Design review of the part built by this model. Coordinates are the model's own, in mm. Face numbers are marked on the shaded views. A direction names the side the tool comes from. Give positions to 0.01 mm unless a question says otherwise; leave off trailing zeros. Write each loop counter-clockwise with the first axis right and the second up, starting at its lowest first coordinate (ties: lowest second). Pieces come first, ordered by that corner, then holes. Notation, with made-up numbers: (51, -16.75) -> (66, -16.75) arc R15 ccw to (66, -5.75) -> close; hole circle Ø5 at (-4, -30.75). An arc over 180 degrees is marked (long way). Answer as a JSON object with one key per item and string values.
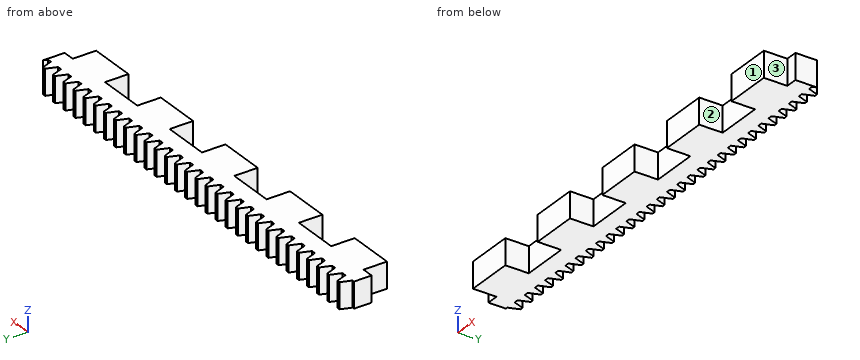
```python
from build123d import *

# Parameters (mm, degrees)
BLANKSKE_W          = 95
BLANKSKE_H          = 11
BLANK_DEPTH         = 5.5
TOOTHCUTSIM_DEPTH   = 96.792745028
TEETHCUTS_COUNT     = 31
TEETHCUTS_PITCH     = 3.14159265
SKETCH_1_W          = 10
SKETCH_1_H          = 5
CUT_EXTRUDE_1_DEPTH = 96.792745028


with BuildPart() as part:
    # BlankSke → Blank (new body)
    with BuildSketch(Plane.XY):
        with Locations((47.5, 5.5)):
            Rectangle(BLANKSKE_W, BLANKSKE_H)
    extrude(amount=-BLANK_DEPTH)

    # TooCutSkeSim → ToothCutSim (cut, through all)
    with BuildSketch(Plane.XY):
        Polygon((0.44443537, 8.75), (-0.44443537, 8.75), (-1.272613241, 11.0254), (1.272613241, 11.0254), align=None)
    toothcutsim = extrude(amount=-TOOTHCUTSIM_DEPTH, mode=Mode.SUBTRACT)

    # TeethCuts: ToothCutSim ×31
    with Locations(*[(i * TEETHCUTS_PITCH, 0, 0) for i in range(1, TEETHCUTS_COUNT)]):
        add(toothcutsim, mode=Mode.SUBTRACT)

    # ｽｹｯﾁ1 → ｶｯﾄ - 押し出し1 (cut, through all)
    with BuildSketch(Plane.XY):
        with Locations((-2.5, 2.5)):
            Rectangle(SKETCH_1_W, SKETCH_1_H)
        with Locations((17.5, 2.5)):
            Rectangle(SKETCH_1_W, SKETCH_1_H)
        with Locations((37.5, 2.5)):
            Rectangle(SKETCH_1_W, SKETCH_1_H)
        with Locations((57.5, 2.5)):
            Rectangle(SKETCH_1_W, SKETCH_1_H)
        with Locations((77.5, 2.5)):
            Rectangle(SKETCH_1_W, SKETCH_1_H)
        with Locations((97.5, 2.5)):
            Rectangle(SKETCH_1_W, SKETCH_1_H)
    extrude(amount=-CUT_EXTRUDE_1_DEPTH, mode=Mode.SUBTRACT)


solid = part.part
```
(1) We need section A-A, the plane y = 3.25. State the section outline as (x, z) points.
Here are the results:
{"outline": "(2.5, -5.5) -> (12.5, -5.5) -> (12.5, 0) -> (2.5, 0) -> close; (22.5, -5.5) -> (32.5, -5.5) -> (32.5, 0) -> (22.5, 0) -> close; (42.5, -5.5) -> (52.5, -5.5) -> (52.5, 0) -> (42.5, 0) -> close; (62.5, -5.5) -> (72.5, -5.5) -> (72.5, 0) -> (62.5, 0) -> close; (82.5, -5.5) -> (92.5, -5.5) -> (92.5, 0) -> (82.5, 0) -> close"}
(2) For line 1 along X through (y, z) = (1.25, -0.6); line 2 along Y through (x, z) = (74, -3.8); line 3 along Y through (x, z) = (28, -1.75), list the stretches that pass through material, from the lowest coordinate up.
Here are the results:
{"line 1": "x = 2.5 to 12.5, 22.5 to 32.5, 42.5 to 52.5, 62.5 to 72.5, 82.5 to 92.5", "line 2": "y = 5 to 11", "line 3": "y = 0 to 8.75"}
(3) Clearance check with flat-ended pins moving along their axes: pin 1 (1.5 mm diameter, centred on y = 2, z = -2.5, fed in from +X); pin 2 (1 mm diameter, centred on y = 6, z = -3, fed in from -X); pin 3 (2 mm diameter, centred on x = 19, z = -5, fed in from -Y). State where each tip first meets the part, or that it passes through.
Here are the results:
{"pin 1": "stops at x = 92.5", "pin 2": "stops at x = 0", "pin 3": "stops at y = 5"}
(4) For the marked faces 1, 2 and 3, list the 3-axis set-ups (+Z, -Z, +X, -X, +Y, -Y) from which the entire face can be reached by the end or side of a thin tool; tool diameter is ignored.
Here are the results:
{"face 1": "+Z, -Z, +X, -X, -Y", "face 2": "+Z, -Z, -Y", "face 3": "+Z, -Z, +X, -Y"}
